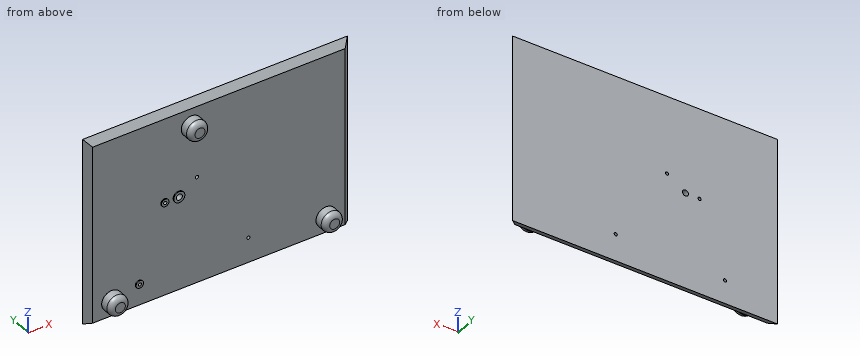
```python
from build123d import *

# Parameters (mm, degrees)
SKETCH3_W           = 260
SKETCH3_H           = 183.5
SKETCH1_W           = 248
SKETCH1_H           = 175
SKETCH1_5_R         = 1.564169695
CUT_EXTRUDE1_DEPTH  = 6
SKETCH1_6_R         = 1.56
SKETCH1_6_R_2       = 2.946919111
CUT_EXTRUDE2_DEPTH  = 6
SKETCH1_7_R         = 1.56
SKETCH1_7_R_2       = 3.675
SKETCH1_7_R_3       = 1.564169695
SKETCH1_7_R_4       = 5.43
SKETCH1_7_R_5       = 2.946919111
BOSS_EXTRUDE2_DEPTH = 1
SKETCH1_9_R         = 1.56
CUT_EXTRUDE9_DEPTH  = 10
SKETCH1_10_R        = 1.563792904
CUT_EXTRUDE11_DEPTH = 10
SKETCH1_11_R        = 9.9
BOSS_EXTRUDE3_DEPTH = 12.5
FILLET1_R           = 5


with BuildPart() as part:
    # Sketch3 → Loft2 section 0
    with BuildSketch(Plane(origin=(0, 6, 0), x_dir=(1, 0, 0), z_dir=(0, 1, 0))):
        with Locations((105.714567309, -62.790792315)):
            Rectangle(SKETCH3_W, SKETCH3_H)
    # Sketch1 → Loft2 section 1
    with BuildSketch(Plane(origin=(0, 0, 0), x_dir=(1, 0, 0), z_dir=(0, 1, 0))):
        with Locations((105.463499551, -60.547933158)):
            Rectangle(SKETCH1_W, SKETCH1_H)
    loft()

    # Sketch1<5> → Cut-Extrude1 (cut)
    with BuildSketch(Plane(origin=(0, 0, 0), x_dir=(1, 0, 0), z_dir=(0, 1, 0))):
        with Locations((52.125403534, -65.240953474)):
            Circle(SKETCH1_5_R)
    extrude(amount=CUT_EXTRUDE1_DEPTH, mode=Mode.SUBTRACT)

    # Sketch1<6> → Cut-Extrude2 (cut)
    with BuildSketch(Plane(origin=(0, 0, 0), x_dir=(1, 0, 0), z_dir=(0, 1, 0))):
        with Locations((27.163499551, 5.952066842)):
            Circle(SKETCH1_6_R)
        with Locations((65.97433474, -65.547933158)):
            Circle(SKETCH1_6_R_2)
    extrude(amount=CUT_EXTRUDE2_DEPTH, mode=Mode.SUBTRACT)

    # Sketch1<7> → Boss-Extrude2 (add)
    with BuildSketch(Plane(origin=(0, 0, 0), x_dir=(1, 0, 0), z_dir=(0, 1, 0))):
        with BuildLine():
            ThreePointArc((30.764919641, 6.683776027), (23.488499551, 5.952066842), (30.764919641, 5.220357657))
            Line((30.764919641, 5.220357657), (30.764919641, 6.683776027))
        make_face()
        with Locations((27.163499551, 5.952066842)):
            Circle(SKETCH1_7_R, mode=Mode.SUBTRACT)
        with Locations((52.125403534, -65.240953474)):
            Circle(SKETCH1_7_R_2)
        with Locations((52.125403534, -65.240953474)):
            Circle(SKETCH1_7_R_3, mode=Mode.SUBTRACT)
        with Locations((65.97433474, -65.547933158)):
            Circle(SKETCH1_7_R_4)
        with Locations((65.97433474, -65.547933158)):
            Circle(SKETCH1_7_R_5, mode=Mode.SUBTRACT)
    extrude(amount=-BOSS_EXTRUDE2_DEPTH)

    # Sketch1<9> → Cut-Extrude9 (cut)
    with BuildSketch(Plane(origin=(0, 0, 0), x_dir=(1, 0, 0), z_dir=(0, 1, 0))):
        with Locations((134.473825947, 2.474049361)):
            Circle(SKETCH1_9_R)
    extrude(amount=CUT_EXTRUDE9_DEPTH, mode=Mode.SUBTRACT)

    # Sketch1<10> → Cut-Extrude11 (cut)
    with BuildSketch(Plane(origin=(0, 0, 0), x_dir=(1, 0, 0), z_dir=(0, 1, 0))):
        with Locations((84.013499551, -77.745508872)):
            Circle(SKETCH1_10_R)
    extrude(amount=CUT_EXTRUDE11_DEPTH, mode=Mode.SUBTRACT)

    # Sketch1<11> → Boss-Extrude3 (add)
    with BuildSketch(Plane(origin=(0, 0, 0), x_dir=(1, 0, 0), z_dir=(0, 1, 0))):
        with Locations((210.683499551, 11.752066842)):
            Circle(SKETCH1_11_R)
        with Locations((78.461853504, -130.95272229)):
            Circle(SKETCH1_11_R)
        with Locations((0.243499551, 11.752066842)):
            Circle(SKETCH1_11_R)
    extrude(amount=-BOSS_EXTRUDE3_DEPTH)

    # Fillet1
    fillet1_edges = [part.edges().sort_by_distance(p)[0] for p in [
        (200.783499551, -12.5, -11.752066842),
        (68.561853504, -12.5, 130.95272229),
        (-9.656500449, -12.5, -11.752066842),
    ]]
    fillet(fillet1_edges, radius=FILLET1_R)


solid = part.part
```
Check sheet for the modelled part. Datum: model origin and axes. Units: mm. Coordinates: 2 decimals unless noted, no trailing zeros. Order: outer loops, then holes, each group sorted by start corner. A loop starts at its lowest first (then second) coordinate and runs counter-clockwise, first axis right, second up. Notation, with made-up numbers: M -16.5,10.5 L 10.5,10.5 A8 ccw 10.5,16.5 Z; hole C -19.5,-9 d3. An arc over 180 degrees is marked long. Write each question's results on one line, items separated by ' | '. Start each with the question number.
1. Cross-section at A-A on y = -4.5. Record the cut outline in (x, z), and give its area (3 significant figures).
2. Material ranges on probe 1 along Y at (x, z) = (101, 19.5); probe 2 along X at (y, z) = (-8, -20); probe 3 along X at (y, z) = (2.25, 144), recorded low to high.
3. Go/stop test with flat-tipped pins: P1, Ø8, axis at x = 27, z = -7, coming from the -Y side; P2, Ø4, axis at x = 134.47, z = -2.47, coming from the +Y side; P3, Ø2, axis at y = -0.5, z = 17, coming from the -X side; P4, Ø6, axis at x = 71, z = 20.5, coming from the -Y side. Record where each tip stops, or that it passes through.
Checks:
1) outline: C 0.24,-11.75 d19.8; C 78.46,130.95 d19.8; C 210.68,-11.75 d19.8 | area: 924 mm²
2) probe 1: y = 0 to 6 | probe 2: x = -5.19 to 5.67, 205.25 to 216.11 | probe 3: x = -20.69 to 231.81
3) P1: stops at y = -1 | P2: stops at y = 6 | P3: stops at x = -19.02 | P4: stops at y = 0
